Here's how the part is built. I have some questions about the finished solid (model axes, mm). Round coordinates to 2 decimals unless told otherwise and drop trailing zeros. Order: outer loops, then holes, each group sorted by start corner. A loop starts at its lowest first (then second) coordinate and runs counter-clockwise, first axis right, second up. Notation, with made-up numbers: (1, -35.5) - (37, -35.5) arc R25 ccw to (37, -2.5) - close; hole circle Ø8 at (40.25, 25.25). An arc over 180 degrees is marked (long way). One line per item, written item: value.
from build123d import *

# Parameters (mm, degrees)
F0_W     = 38.1
F0_H     = 19.05
F0_R     = 2
F0_W_2   = 30
F0_H_2   = 53.175
F1_DEPTH = 5
F2_SIZE  = 19.05
F4_DEPTH = 5.001
F5_DEPTH = 25.4
F6_SIZE  = 12.7


with BuildPart() as f1:
    # F0 (on Front) → F1 (new body)
    with BuildSketch(Plane.XZ):
        with Locations((34.05, 0)):
            Rectangle(F0_W, F0_H)
        with Locations((43.1, 0)):
            Circle(F0_R, mode=Mode.SUBTRACT)
        with Locations((0, 36.1125)):
            Rectangle(F0_W_2, F0_H_2)
        with Locations((-34.05, 0)):
            Rectangle(F0_W, F0_H)
        with Locations((-43.1, 0)):
            Circle(F0_R, mode=Mode.SUBTRACT)
        Rectangle(F0_W_2, F0_H)
    extrude(amount=F1_DEPTH)

    # F2
    f2_edges = [f1.edges().sort_by_distance(p)[0] for p in [
        (15, -2.5, 9.525),
        (-15, -2.5, 9.525),
    ]]
    chamfer(f2_edges, length=F2_SIZE)

    # F3 (on face) → F4 (cut, through all)
    with BuildSketch(Plane.XZ.offset(5)):
        Polygon((-8, 52.025), (8, 52.025), (8, 11.525), (8, 9.525), (34.05, 9.525), (15, 28.575), (15, 62.7), (-15, 62.7), (-15, 28.575), (-34.05, 9.525), (-8, 9.525), (-8, 11.525), align=None)
    extrude(amount=-F4_DEPTH, mode=Mode.SUBTRACT)

    # F3 (on face) → F5 (cut)
    with BuildSketch(Plane.XZ.offset(5)):
        with BuildLine():
            ThreePointArc((0, 42.025), (1.4142135624, 42.6107864376), (2, 44.025))
            ThreePointArc((2, 44.025), (-1.4142135624, 45.4392135624), (0, 42.025))
        make_face()
        with BuildLine():
            ThreePointArc((2, 19.525), (1.4142135624, 20.9392135624), (0, 21.525))
            ThreePointArc((0, 21.525), (-1.4142135624, 18.1107864376), (2, 19.525))
        make_face()
    extrude(amount=-F5_DEPTH, mode=Mode.SUBTRACT)

    # F6
    f6_edges = [f1.edges().sort_by_distance(p)[0] for p in [
        (8, -2.5, 9.525),
        (-8, -2.5, 9.525),
    ]]
    chamfer(f6_edges, length=F6_SIZE)


solid = f1.part
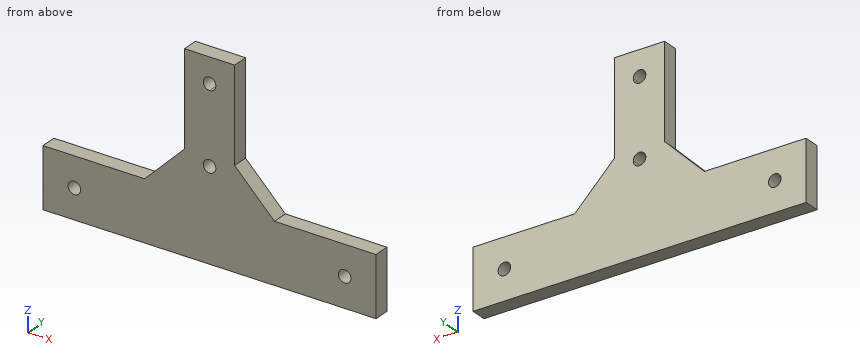
Q1. If we section it at D-D, the plane x = 43.5: Please give me the cut outline in (y, z) (3 decimals), then the cut area to 3 significant figures.
Results list:
outline: (-5, -9.525) - (0, -9.525) - (0, -1.96) - (-5, -1.96) - close; (-5, 1.96) - (0, 1.96) - (0, 9.525) - (-5, 9.525) - close
area: 75.7 mm²
Q2. If I drill on line 1 along Z through (x, y) = (43.1, -3.3) (3 decimals); line 2 along Z through (x, y) = (-38.5, -4.45) (3 decimals); line 3 along X through (y, z) = (-3.8, 49.5), over which ranges is the centre line in solid material (lowest first)?
Results list:
line 1: -9.525 to -2, 2 to 9.525
line 2: -9.525 to 9.525
line 3: -8 to 8
Q3. If we section it at C-C, the plane y = -2.5: Please give me the cut outline in (x, z) (3 decimals), then the cut area to 3 significant figures.
Results list:
outline: (-53.1, -9.525) - (53.1, -9.525) - (53.1, 9.525) - (20.7, 9.525) - (8, 22.225) - (8, 52.025) - (-8, 52.025) - (-8, 22.225) - (-20.7, 9.525) - (-53.1, 9.525) - close; hole circle Ø4 at (-43.1, 0); hole circle Ø4 at (0, 19.525); hole circle Ø4 at (0, 44.025); hole circle Ø4 at (43.1, 0)
area: 2,810 mm²
Q4. If we section it at B-B, the plane x = -43.1: Please give me the cut outline in (y, z) (3 decimals), then the cut area to 4 significant figures.
Results list:
outline: (-5, -9.525) - (0, -9.525) - (0, -2) - (-5, -2) - close; (-5, 2) - (0, 2) - (0, 9.525) - (-5, 9.525) - close
area: 75.25 mm²
Q5. Will these pins go through, and if not, where does the flat tip stop? pin 1 (1.5 mm diameter, centred on x = 30, y = -3, fed in from +Z) (3 decimals); pin 2 (3.5 mm diameter, centred on x = -43.1, z = 0, fed in from +Y).
Results list:
pin 1: z = 9.525
pin 2: through
Q6. If we section it at A-A, the plane z = 0: Please give me the cut outline in (x, y), then the cut area to 3 significant figures.
Results list:
outline: (-53.1, -5) - (-45.1, -5) - (-45.1, 0) - (-53.1, 0) - close; (-41.1, -5) - (41.1, -5) - (41.1, 0) - (-41.1, 0) - close; (45.1, -5) - (53.1, -5) - (53.1, 0) - (45.1, 0) - close
area: 491 mm²
